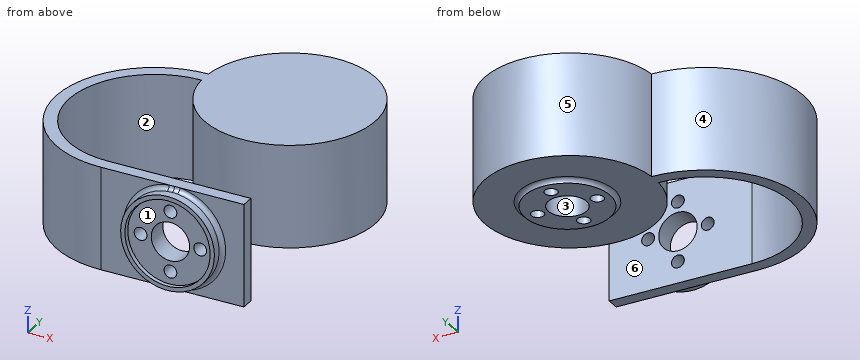
```python
from build123d import *

# Parameters (mm, degrees)
BOSS_EXTRUDE1_DEPTH = 24
SKETCH2_R           = 10
BOSS_EXTRUDE2_DEPTH = 2
SKETCH3_R           = 1.5
SKETCH3_R_2         = 4.5
CUT_EXTRUDE1_DEPTH  = 5
SKETCH6_R           = 10
BOSS_EXTRUDE3_DEPTH = 1
FILLET2_R           = 1
SKETCH7_R           = 1.5
SKETCH7_R_2         = 4.5
CUT_EXTRUDE4_DEPTH  = 10
SKETCH9_R           = 11
SKETCH9_R_2         = 10
BOSS_EXTRUDE4_DEPTH = 3
FILLET3_R           = 1


with BuildPart() as part:
    # Sketch1 → Boss-Extrude1 (new body)
    with BuildSketch(Plane.XY):
        with BuildLine():
            Line((30.263122148, -52.276236142), (30.263122148, -49.276236142))
            Line((30.263122148, -49.276236142), (-3.247333847, -49.276236142))
            ThreePointArc((-3.247333847, -49.276236142), (-23.247333847, -29.276236142), (-3.247333847, -9.276236142))
            ThreePointArc((-3.247333847, -9.276236142), (36.696336828, -7.776236142), (-3.247333847, -6.276236142))
            ThreePointArc((-3.247333847, -6.276236142), (-26.247333847, -29.276236142), (-3.247333847, -52.276236142))
            Line((-3.247333847, -52.276236142), (30.263122148, -52.276236142))
        make_face()
    extrude(amount=BOSS_EXTRUDE1_DEPTH)

    # Sketch2 → Boss-Extrude2 (add)
    with BuildSketch(Plane.XZ.offset(52.276236142)):
        with Locations(Location((14.119877924, 12.054461488, 0), (0, 0, 90))):
            Circle(SKETCH2_R)
    extrude(amount=BOSS_EXTRUDE2_DEPTH)

    # Sketch3 → Cut-Extrude1 (cut)
    with BuildSketch(Plane.XZ.offset(54.276236142)):
        with Locations(Location((14.119877924, 19.054461488, 0), (0, 0, 270))):
            Circle(SKETCH3_R)
        with Locations(Location((21.119877924, 12.054461488, 0), (0, 0, 270))):
            Circle(SKETCH3_R)
        with Locations(Location((14.119877924, 5.054461488, 0), (0, 0, 270))):
            Circle(SKETCH3_R)
        with Locations(Location((7.119877924, 12.054461488, 0), (0, 0, 270))):
            Circle(SKETCH3_R)
        with Locations(Location((14.119877924, 12.054461488, 0), (0, 0, 270))):
            Circle(SKETCH3_R_2)
    extrude(amount=-CUT_EXTRUDE1_DEPTH, mode=Mode.SUBTRACT)

    # Sketch6 → Boss-Extrude3 (add)
    with BuildSketch(Plane(origin=(0, 0, 0), x_dir=(-1, 0, 0), z_dir=(0, 0, -1))):
        with Locations((-17.221710812, -7.598312744)):
            Circle(SKETCH6_R)
    extrude(amount=BOSS_EXTRUDE3_DEPTH)

    # Fillet2
    fillet2_edges = [part.edges().sort_by_distance(p)[0] for p in [
        (27.221710812, -7.598312744, 0),
    ]]
    fillet(fillet2_edges, radius=FILLET2_R - 0.0001)  # a hair under: the kernel refuses the full size

    # Sketch7 → Cut-Extrude4 (cut)
    with BuildSketch(Plane(origin=(0, 0, -1), x_dir=(-1, 0, 0), z_dir=(0, 0, -1))):
        with Locations((-17.221710812, -0.598312744)):
            Circle(SKETCH7_R)
        with Locations((-10.221710812, -7.598312744)):
            Circle(SKETCH7_R)
        with Locations((-17.221710812, -14.598312744)):
            Circle(SKETCH7_R)
        with Locations((-24.221710812, -7.598312744)):
            Circle(SKETCH7_R)
        with Locations((-17.221710812, -7.598312744)):
            Circle(SKETCH7_R_2)
    extrude(amount=-CUT_EXTRUDE4_DEPTH, mode=Mode.SUBTRACT)

    # Sketch9 → Boss-Extrude4 (add)
    with BuildSketch(Plane.XZ.offset(52.276236142)):
        with Locations(Location((13.990564712, 12.070439632, 0), (0, 0, 90))):
            Circle(SKETCH9_R)
        with Locations(Location((13.990564712, 12.070439632, 0), (0, 0, 82.582870782))):
            Circle(SKETCH9_R_2, mode=Mode.SUBTRACT)
    extrude(amount=BOSS_EXTRUDE4_DEPTH)

    # Fillet3
    fillet3_edges = [part.edges().sort_by_distance(p)[0] for p in [
        (13.990564712, -52.276236142, 1.070439632),
    ]]
    fillet(fillet3_edges, radius=FILLET3_R)


solid = part.part
```
The model under review builds one solid part; all positions refer to its coordinate system, in mm. Face numbers are marked on the shaded views. A direction names the side the tool comes from. Coordinates: 2 decimals unless noted, no trailing zeros. Write each loop counter-clockwise with the first axis right and the second up, starting at its lowest first coordinate (ties: lowest second). Pieces come first, ordered by that corner, then holes.
1) We need section B-B on z = 12. Count the separate pieces of the cut face and the enclosed holes in it, then the cut area to 3 significant figures.
2) We need section A-A on x = 1. State the section outline as (y, z) points, then the cut area to 3 significant figures.
3) Clearance check with flat-ended pins moving along their axes: pin 1 Ø1 at (x, z) = (2.5, 20) entering from +Y; pin 2 Ø8 at (x, z) = (-13.5, 17.5) entering from +Y; pin 3 Ø2 at (x, z) = (15.5, 13.5) entering from +Y; pin 4 Ø3.5 at (x, y) = (17.5, 0) entering from -Z. State where each tip first meets the part, or that it passes through.
4) We need section C-C on y = -30.5. State the section outline as (x, z) points.
5) We need section D-D on y = 4.5. State the section outline as (x, z) points.
6) Machinability: for the marked faces 1, 2 and 3, which of the approach directions +Z, -Z, +X, -X, +Y, -Y give a long, thin tool a straight path to every point of the face, cutting with its end or side? Answer none if there is none.
7) The part is to be moulded in two halves that separate along X. For the marked faces 4, 5 and 6, say which applies: pulls with the +X half, pulls with the -X half, needs draft (parallel to the pull), parting line crosses it, or undercut.
8) To check wall thickness, follow probe 1 along Y at (x, z) = (16, 22.25); probe 2 along X at (y, z) = (-13.5, 8); probe 3 along Z at (x, y) = (29, -4). State the ranges of each line that lie inside material, in increasing order.
Answer list:
1. separate pieces: 4
1. enclosed holes: 0
1. area: 1,530 mm2
2. outline: (-52.28, 0) - (-49.28, 0) - (-49.28, 24) - (-52.28, 24) - close; (-20.17, 0) - (4.62, 0) - (4.62, 24) - (-20.17, 24) - close
2. area: 667 mm2
3. pin 1: stops at y = 6.8
3. pin 2: stops at y = -7.14
3. pin 3: stops at y = 12.22
3. pin 4: stops at z = -1
4. outline: (-26.21, 0) - (-23.21, 0) - (-23.21, 24) - (-26.21, 24) - close
5. outline: (0.91, 0) - (32.49, 0) - (32.49, 24) - (0.91, 24) - close
6. face 1: -Y
6. face 2: +Z, -Z
6. face 3: -Z
7. face 4: pulls with the -X half
7. face 5: undercut
7. face 6: needs draft
8. probe 1: y = -55.28 to -49.28, -27.76 to 12.21
8. probe 2: x = -19.98 to -15.54, -2.47 to 16.2, 18.24 to 35.86
8. probe 3: z = 0 to 24
